from build123d import *

# Parameters (mm, degrees)
SKETCH1_W           = 160.02
SKETCH1_H           = 65.151
BOSS_EXTRUDE1_DEPTH = 5.461
SKETCH2_W           = 5.461
SKETCH2_H           = 15.875
CUT_EXTRUDE1_DEPTH  = 6.461
SKETCH4_W           = 19.05
SKETCH4_H           = 5.461
BOSS_EXTRUDE3_DEPTH = 5.461


with BuildPart() as part:
    # Sketch1 → Boss-Extrude1 (new body)
    with BuildSketch(Plane.XY):
        Rectangle(SKETCH1_W, SKETCH1_H)
    extrude(amount=BOSS_EXTRUDE1_DEPTH)

    # Sketch2 → Cut-Extrude1 (cut, through all)
    with BuildSketch(Plane.XY.offset(5.461)):
        with Locations((-77.2795, 24.638)):
            Rectangle(SKETCH2_W, SKETCH2_H)
        with Locations((-77.2795, -24.638)):
            Rectangle(SKETCH2_W, SKETCH2_H)
        with Locations((77.2795, 24.638)):
            Rectangle(SKETCH2_W, SKETCH2_H)
        with Locations((77.2795, -24.638)):
            Rectangle(SKETCH2_W, SKETCH2_H)
    extrude(amount=-CUT_EXTRUDE1_DEPTH, mode=Mode.SUBTRACT)

    # Sketch4 → Boss-Extrude3 (add)
    with BuildSketch(Plane.XY.offset(5.461)):
        with Locations((-57.785, 35.306)):
            Rectangle(SKETCH4_W, SKETCH4_H)
        with Locations((-57.785, -35.306)):
            Rectangle(SKETCH4_W, SKETCH4_H)
    extrude(amount=-BOSS_EXTRUDE3_DEPTH)


solid = part.part
CAD build for the part. Positions are in the model's coordinates, mm. A direction names the side the tool comes from. Give positions to 0.01 mm unless a question says otherwise; leave off trailing zeros. Write each loop counter-clockwise with the first axis right and the second up, starting at its lowest first coordinate (ties: lowest second). Pieces come first, ordered by that corner, then holes. Notation, with made-up numbers: (58, 14) -> (100, 14) arc R23 ccw to (100, 29) -> close; hole circle Ø7 at (27, -21.5). An arc over 180 degrees is marked (long way). Return JSON: item names as keys, results as strings.
Item 1: Band-saw the part on B-B (y = -27). List the corners of the cut face in (x, z), then the cut area to 3 significant figures.
Answer below:
{"outline": "(-74.55, 0) -> (74.55, 0) -> (74.55, 5.46) -> (-74.55, 5.46) -> close", "area": "814 mm2"}
Item 2: Band-saw the part on C-C (x = 48.5). List the corners of the cut face in (y, z).
Answer below:
{"outline": "(-32.58, 0) -> (32.58, 0) -> (32.58, 5.46) -> (-32.58, 5.46) -> close"}
Item 3: Drill centre lines: probe 1 along X at (y, z) = (-19.5, 2.45); probe 2 along Y at (x, z) = (-40, 1); probe 3 along X at (y, z) = (34, 1.5). Where is each one in solid material? Low to high.
Answer below:
{"probe 1": "x = -74.55 to 74.55", "probe 2": "y = -32.58 to 32.58", "probe 3": "x = -67.31 to -48.26"}
Item 4: Tool access for faces 1 (the flat face through (12, 32.575, 3)), 2 (the flat face through (-77, 16.7, 3)), 3 (the flat face through (77, -16.7, 3)): list every direction of +Z, -Z, +X, -X, +Y, -Y with a clear straight run to the whole face (end or side of a thin tool).
Answer below:
{"face 1": "+Z, -Z, +X, +Y", "face 2": "+Z, -Z, -X, +Y", "face 3": "+Z, -Z, +X, -Y"}
Item 5: Drop flat-ended pins along their axis: pin 1 (1.6 mm diameter, centred on y = -36, z = 2.5, fed in from -X); pin 2 (2.5 mm diameter, centred on x = 78, z = 1.5, fed in from -Y); pin 3 (1.5 mm diameter, centred on x = 10.5, z = 0.5, fed in from -Y). Give the stop position or say it passes through.
Answer below:
{"pin 1": "stops at x = -67.31", "pin 2": "stops at y = -16.7", "pin 3": "stops at y = -32.58"}
Item 6: Band-saw the part on A-A (z = 4.6). List the corners of the cut face in (x, y), then the cut area to 3 significant figures.
Answer below:
{"outline": "(-80.01, -16.7) -> (-74.55, -16.7) -> (-74.55, -32.58) -> (-67.31, -32.58) -> (-67.31, -38.04) -> (-48.26, -38.04) -> (-48.26, -32.58) -> (74.55, -32.58) -> (74.55, -16.7) -> (80.01, -16.7) -> (80.01, 16.7) -> (74.55, 16.7) -> (74.55, 32.58) -> (-48.26, 32.58) -> (-48.26, 38.04) -> (-67.31, 38.04) -> (-67.31, 32.58) -> (-74.55, 32.58) -> (-74.55, 16.7) -> (-80.01, 16.7) -> close", "area": "10,300 mm2"}
